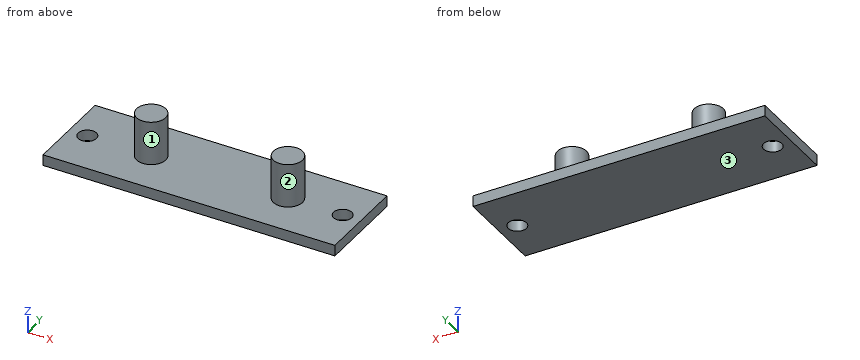
from build123d import *

# Parameters (mm, degrees)
SKETCH1_W           = 80
SKETCH1_H           = 25
BOSS_EXTRUDE1_DEPTH = 3
SKETCH2_R           = 4
BOSS_EXTRUDE2_DEPTH = 12
SKETCH3_R           = 2.5
CUT_EXTRUDE1_DEPTH  = 8


with BuildPart() as part:
    # Sketch1 → Boss-Extrude1 (new body)
    with BuildSketch(Plane.XY):
        with Locations((-40, 12.5)):
            Rectangle(SKETCH1_W, SKETCH1_H)
    extrude(amount=BOSS_EXTRUDE1_DEPTH)

    # Sketch2 → Boss-Extrude2 (add)
    with BuildSketch(Plane.XY.offset(3)):
        with Locations((-57.5, 12.5)):
            Circle(SKETCH2_R)
        with Locations((-20, 12.5)):
            Circle(SKETCH2_R)
    extrude(amount=BOSS_EXTRUDE2_DEPTH)

    # Sketch3 → Cut-Extrude1 (cut)
    with BuildSketch(Plane.XY.offset(3)):
        with Locations((-75, 12.5)):
            Circle(SKETCH3_R)
        with Locations((-5, 12.5)):
            Circle(SKETCH3_R)
    extrude(amount=-CUT_EXTRUDE1_DEPTH, mode=Mode.SUBTRACT)


solid = part.part
Here's how the part is built. I have some questions about the finished solid (model axes, mm). Face numbers are marked on the shaded views. Coordinates: 2 decimals unless noted, no trailing zeros. Order: outer loops, then holes, each group sorted by start corner. A loop starts at its lowest first (then second) coordinate and runs counter-clockwise, first axis right, second up. Notation, with made-up numbers: (-8, 20) -> (43, 20) arc R25 ccw to (43, 57) -> close; hole circle Ø5 at (-26, -34.5). An arc over 180 degrees is marked (long way). Answer in a Markdown table with one row per item.
(1) I want a section at D-D on x = -20. List the corners of the cut face in (y, z) for me.
Answer key:
| item | result |
|---|---|
| outline | (0, 0) -> (25, 0) -> (25, 3) -> (16.5, 3) -> (16.5, 15) -> (8.5, 15) -> (8.5, 3) -> (0, 3) -> close |
(2) I want a section at B-B on y = 13.5. List the corners of the cut face in (x, z) for me.
Answer key:
| item | result |
|---|---|
| outline | (-80, 0) -> (-77.29, 0) -> (-77.29, 3) -> (-80, 3) -> close; (-72.71, 0) -> (-7.29, 0) -> (-7.29, 3) -> (-16.13, 3) -> (-16.13, 15) -> (-23.87, 15) -> (-23.87, 3) -> (-53.63, 3) -> (-53.63, 15) -> (-61.37, 15) -> (-61.37, 3) -> (-72.71, 3) -> close; (-2.71, 0) -> (0, 0) -> (0, 3) -> (-2.71, 3) -> close |
(3) I want a section at A-A on x = -5. List the corners of the cut face in (y, z) for me.
Answer key:
| item | result |
|---|---|
| outline | (0, 0) -> (10, 0) -> (10, 3) -> (0, 3) -> close; (15, 0) -> (25, 0) -> (25, 3) -> (15, 3) -> close |
(4) Will these pins go through, and if not, where does the flat tip stop? pin 1 Ø6.5 at (x, y) = (-5, 12.5) entering from +Z; pin 2 Ø3 at (x, y) = (-75, 12.5) entering from +Z; pin 3 Ø5 at (x, z) = (-18.5, 13) entering from -Y.
Answer key:
| item | result |
|---|---|
| pin 1 | z = 3 |
| pin 2 | through |
| pin 3 | y = 8.5 |
(5) Thinking about a two-plate mould opening in X: for the marked faces 1, 2 and 3, which applies, +X half, -X half, draft (parallel to the pull), parting line (faces both ways), or undercut?
Answer key:
| item | result |
|---|---|
| face 1 | undercut |
| face 2 | undercut |
| face 3 | draft |
(6) Please list where these lines run through material, in increasing order: probe 1 along Y at (x, z) = (-5, 2.2); probe 2 along X at (y, z) = (11.25, 1.25); probe 3 along Z at (x, y) = (-14.5, 22.5).
Answer key:
| item | result |
|---|---|
| probe 1 | 0 to 10, 15 to 25 |
| probe 2 | -80 to -77.17, -72.83 to -7.17, -2.83 to 0 |
| probe 3 | 0 to 3 |
(7) I want a section at C-C on z = 1.75. List the corners of the cut face in (x, y) for me, then the cut area to 3 significant figures.
Answer key:
| item | result |
|---|---|
| outline | (-80, 0) -> (0, 0) -> (0, 25) -> (-80, 25) -> close; hole circle Ø5 at (-75, 12.5); hole circle Ø5 at (-5, 12.5) |
| area | 1,960 mm^2 |
